Read the model definition and answer for the solid it produces. Units are mm, in the model's axes. A direction names the side the tool comes from. Round coordinates to 2 decimals unless told otherwise and drop trailing zeros. Write each loop counter-clockwise with the first axis right and the second up, starting at its lowest first coordinate (ties: lowest second). Pieces come first, ordered by that corner, then holes.
from build123d import *

# Parameters (mm, degrees)
SKETCH_1_W          = 4
SKETCH_1_H          = 6
EXTRUDE_1_DEPTH     = 25
SKETCH_3_W          = 1.5
SKETCH_3_H          = 1
CUT_EXTRUDE_1_DEPTH = 10


with BuildPart() as part:
    # 草图1 → 凸台-拉伸1 (new body)
    with BuildSketch(Plane(origin=(0, 0, 0), x_dir=(0, 0, -1), z_dir=(1, 0, 0))):
        with Locations((0, 3)):
            Rectangle(SKETCH_1_W, SKETCH_1_H)
    extrude(amount=EXTRUDE_1_DEPTH)

    # 草图3 → 切除-拉伸1 (cut, symmetric)
    with BuildSketch(Plane.XY):
        with Locations((5.25, 0.5)):
            Rectangle(SKETCH_3_W, SKETCH_3_H)
        with Locations((5.25, 5.5)):
            Rectangle(SKETCH_3_W, SKETCH_3_H)
        with Locations((19.75, 5.5)):
            Rectangle(SKETCH_3_W, SKETCH_3_H)
        with Locations((19.75, 0.5)):
            Rectangle(SKETCH_3_W, SKETCH_3_H)
    extrude(amount=CUT_EXTRUDE_1_DEPTH, both=True, mode=Mode.SUBTRACT)


solid = part.part
Q1. Straight lines are drawn through the part: probe 1 along X at (y, z) = (0.8, -1.4); probe 2 along Y at (x, z) = (5.25, 0.25). For each, find the intervals that lie inside material, in ascending order.
Verdict:
probe 1: x = 0 to 4.5, 6 to 19, 20.5 to 25
probe 2: y = 1 to 5
Q2. Determine the mould class of faces 4 (the flat face through (0, 3, 0)), 5 (the flat face through (4.5, 0.5, 0)), 6 (the flat face through (20, 5, 0)), 7 (the flat face through (23, 0, 0)) for opening direction X: pulls with the +X half, pulls with the -X half, needs draft (parallel to the pull), parting line crosses it, or undercut.
Verdict:
face 4: pulls with the -X half
face 5: undercut
face 6: undercut
face 7: needs draft
Q3. Flat-ended cylindrical pins translate along their axes: pin 1 Ø1.2 at (x, z) = (5, -0.5) entering from -Y; pin 2 Ø0.8 at (x, z) = (5, 1) entering from +Y. Find the tip coordinate at first contact, or state that the pin passes through.
Verdict:
pin 1: stops at y = 0
pin 2: stops at y = 5
Q4. Section A-A (z = -0.6) is taken. Determine the outline of the cut face in (x, y), then the cut area to 3 significant figures.
Verdict:
outline: (0, 0) - (4.5, 0) - (4.5, 1) - (6, 1) - (6, 0) - (19, 0) - (19, 1) - (20.5, 1) - (20.5, 0) - (25, 0) - (25, 6) - (20.5, 6) - (20.5, 5) - (19, 5) - (19, 6) - (6, 6) - (6, 5) - (4.5, 5) - (4.5, 6) - (0, 6) - close
area: 144 mm2
Q5. Which of the six approach directions +Z, -Z, +X, -X, +Y, -Y give full straight-line access (tool end or side, diameter ignored) to faces 1 (the flat face through (20.5, 5.5, 0)), 2 (the flat face through (2, 6, 0)), 3 (the flat face through (5, 1, 0))?
Verdict:
face 1: +Z, -Z, +Y
face 2: +Z, -Z, +X, -X, +Y
face 3: +Z, -Z, -Y
